```python
from build123d import *

# Parameters (mm, degrees)
F0_W     = 60
F0_H     = 80
F0_R     = 2.75
F1_DEPTH = 2
F2_W     = 30
F2_H     = 30
F2_W_2   = 26
F2_H_2   = 26
F3_DEPTH = 1002
F4_R     = 5
F5_DEPTH = 5
F6_W     = 40
F6_H     = 40
F6_R     = 3.5
F6_W_2   = 30
F7_DEPTH = 2
F6_R_2   = 5
F8_DEPTH = 5


with BuildPart() as f1:
    # F0 (on Front) → F1 (new body)
    with BuildSketch(Plane.XZ):
        Rectangle(F0_W, F0_H)
        with Locations((-24, -34)):
            Circle(F0_R, mode=Mode.SUBTRACT)
        with Locations((24, -34)):
            Circle(F0_R, mode=Mode.SUBTRACT)
        with Locations((-24, 34)):
            Circle(F0_R, mode=Mode.SUBTRACT)
        with Locations((24, 34)):
            Circle(F0_R, mode=Mode.SUBTRACT)
    extrude(amount=F1_DEPTH)

    # F2 (on Front) → F3 (join)
    with BuildSketch(Plane.XZ):
        Rectangle(F2_W, F2_H)
        Rectangle(F2_W_2, F2_H_2, mode=Mode.SUBTRACT)
    extrude(amount=F3_DEPTH)

    # F4 (on face) → F5 (cut)
    with BuildSketch(Plane.XY.offset(15)):
        with Locations((0, -15.7746840268)):
            Circle(F4_R)
    extrude(amount=-F5_DEPTH, mode=Mode.SUBTRACT)

    # F6 (on face) → F7 (join)
    with BuildSketch(Plane(origin=(0, 0, -15), x_dir=(1, 0, 0), z_dir=(0, 0, -1))):
        with Locations((35, 982)):
            Rectangle(F6_W, F6_H)
        with Locations((35, 982)):
            Circle(F6_R, mode=Mode.SUBTRACT)
        with Locations((0, 982)):
            Rectangle(F6_W_2, F6_H)
        with Locations((-35, 982)):
            Rectangle(F6_W, F6_H)
        with Locations((-34.9994153271, 982.2861011526)):
            Circle(F6_R, mode=Mode.SUBTRACT)
    extrude(amount=F7_DEPTH)

    # F6 (on face) → F8 (cut)
    with BuildSketch(Plane(origin=(0, 0, -15), x_dir=(1, 0, 0), z_dir=(0, 0, -1))):
        with Locations((0, 939.2803311348)):
            Circle(F6_R_2)
    extrude(amount=-F8_DEPTH, mode=Mode.SUBTRACT)


solid = f1.part
```
Here's how the part is built. I have some questions about the finished solid (model axes, mm). A direction names the side the tool comes from. Round coordinates to 2 decimals unless told otherwise and drop trailing zeros. Order: outer loops, then holes, each group sorted by start corner. A loop starts at its lowest first (then second) coordinate and runs counter-clockwise, first axis right, second up. Notation, with made-up numbers: (-10, -20.5) -> (35, -20.5) arc R34 ccw to (35, 10.5) -> close; hole circle Ø11 at (-20.75, 4.25). An arc over 180 degrees is marked (long way). Use a Markdown table: item, result. Add a question column.
(1) For pin 1 Ø3 at (y, z) = (-284.5, 13) entering from -X; pin 2 Ø8 at (y, z) = (-687, -4.5) entering from +X; pin 3 Ø2 at (y, z) = (-0.5, -16.5) entering from +X; pin 4 Ø4 at (x, y) = (35, -982) entering from -Z, each with a flat end and sliding along its axis, tell me the tip position at first contact or that it passes through.
(2) I need wall thicknesses on line 1 along Z through (x, y) = (24, -1); line 2 along X through (y, z) = (-982, -15.65); line 3 along X through (y, z) = (-240, 2). Which ranges of each line are inside material? Lowest first, please.
(3) Suppose I cut it at A-A, the plane y = -108.5. Please give me the cut outline in (x, z).
(4) If we mould it in two halves opening along Z, with no side actions, what happens to faces 6 (the face through (0, 0, 1)), 7 (the face through (0, -495, 13)), 8 (the face through (-1, -982, -17))? For each: released by +Z, released by -Z, zero draft, split by the parting line, or undercut.
(5) For faces 1 (the face through (0, -475, -15)), 2 (the face through (-35, -987, -15)), 3 (the face through (35, -987, -15)), 4 (the face through (0, -495, -13)), 5 (the face through (0, -495, 15)), which set-ups out of +Z, -Z, +X, -X, +Y, -Y let a thin tool reach every point of the face, with its end or its side?
Verdict:
| question | item | result |
|---|---|---|
| 1 | pin 1 | x = -15 |
| 1 | pin 2 | x = 15 |
| 1 | pin 3 | x = 30 |
| 1 | pin 4 | through |
| 2 | line 1 | -40 to -36.75, -31.25 to 31.25, 36.75 to 40 |
| 2 | line 2 | -55 to -38.49, -31.51 to 31.5, 38.5 to 55 |
| 2 | line 3 | -15 to -13, 13 to 15 |
| 3 | outline | (-15, -15) -> (15, -15) -> (15, 15) -> (-15, 15) -> close; hole (-13, -13) -> (13, -13) -> (13, 13) -> (-13, 13) -> close |
| 4 | face 6 | zero draft |
| 4 | face 7 | undercut |
| 4 | face 8 | released by -Z |
| 5 | face 1 | -Z, +X, -X |
| 5 | face 2 | +Z, -X, -Y |
| 5 | face 3 | +Z, +X, -Y |
| 5 | face 4 | -Y |
| 5 | face 5 | +Z, +X, -X, -Y |
